The model under review builds one solid part; all positions refer to its coordinate system, in mm. A direction names the side the tool comes from. Coordinates: 2 decimals unless noted, no trailing zeros. Order: outer loops, then holes, each group sorted by start corner. A loop starts at its lowest first (then second) coordinate and runs counter-clockwise, first axis right, second up. Notation, with made-up numbers: (-24.75, 89) -> (12.25, 89) arc R11 ccw to (12.25, 93) -> close; hole circle Ø1 at (76, -19). An arc over 180 degrees is marked (long way). Put each result on its own line as item: value.
from build123d import *

# Parameters (mm, degrees)
F0_R     = 5
F1_DEPTH = 10


with BuildPart() as f1:
    # F0 (on Top) → F1 (new body)
    with BuildSketch(Plane.XY):
        with BuildLine():
            Line((-14.934364, 27.165507), (-14.585732, 20.304099))
            ThreePointArc((-14.585732, 20.304099), (-14.694631, 20.225425), (-14.803106, 20.146167))
            Line((-14.803106, 20.146167), (-21.22096, 22.598027))
            Line((-21.22096, 22.598027), (-19.176918, 16.038884))
            ThreePointArc((-19.176918, 16.038884), (-19.262831, 15.9356), (-19.348188, 15.831855))
            Line((-19.348188, 15.831855), (-26.174166, 16.610631))
            Line((-26.174166, 16.610631), (-22.563148, 10.765888))
            ThreePointArc((-22.563148, 10.765888), (-22.620676, 10.644482), (-22.677551, 10.52277))
            Line((-22.677551, 10.52277), (-29.482752, 9.579527))
            Line((-29.482752, 9.579527), (-24.531653, 4.816431))
            ThreePointArc((-24.531653, 4.816431), (-24.557181, 4.684533), (-24.582, 4.5525))
            Line((-24.582, 4.5525), (-30.938829, 1.946506))
            Line((-30.938829, 1.946506), (-24.958744, -1.43566))
            ThreePointArc((-24.958744, -1.43566), (-24.950668, -1.569763), (-24.941872, -1.70382))
            Line((-24.941872, -1.70382), (-30.450905, -5.808821))
            Line((-30.450905, -5.808821), (-23.817584, -7.597544))
            ThreePointArc((-23.817584, -7.597544), (-23.776413, -7.725425), (-23.734555, -7.853083))
            Line((-23.734555, -7.853083), (-28.049639, -13.199158))
            Line((-28.049639, -13.199158), (-21.179879, -13.282045))
            ThreePointArc((-21.179879, -13.282045), (-21.108198, -13.39567), (-21.035908, -13.508908))
            Line((-21.035908, -13.508908), (-23.885911, -19.760144))
            Line((-23.885911, -19.760144), (-17.211364, -18.131987))
            ThreePointArc((-17.211364, -18.131987), (-17.113678, -18.224216), (-17.015497, -18.315918))
            Line((-17.015497, -18.315918), (-18.221343, -25.079527))
            Line((-18.221343, -25.079527), (-12.161395, -21.84263))
            ThreePointArc((-12.161395, -21.84263), (-12.043842, -21.907667), (-11.925941, -21.972072))
            Line((-11.925941, -21.972072), (-11.411861, -28.823071))
            Line((-11.411861, -28.823071), (-6.347282, -24.180819))
            ThreePointArc((-6.347282, -24.180819), (-6.217247, -24.214579), (-6.087033, -24.24764))
            Line((-6.087033, -24.24764), (-3.88533, -30.755556))
            Line((-3.88533, -30.755556), (-0.134345, -24.999639))
            ThreePointArc((-0.134345, -24.999639), (0, -25), (0.134345, -24.999639))
            Line((0.134345, -24.999639), (3.88533, -30.755556))
            Line((3.88533, -30.755556), (6.087033, -24.24764))
            ThreePointArc((6.087033, -24.24764), (6.217247, -24.214579), (6.347282, -24.180819))
            Line((6.347282, -24.180819), (11.411861, -28.823071))
            Line((11.411861, -28.823071), (11.925941, -21.972072))
            ThreePointArc((11.925941, -21.972072), (12.043842, -21.907667), (12.161395, -21.84263))
            Line((12.161395, -21.84263), (18.221343, -25.079527))
            Line((18.221343, -25.079527), (17.015497, -18.315918))
            ThreePointArc((17.015497, -18.315918), (17.113678, -18.224216), (17.211364, -18.131987))
            Line((17.211364, -18.131987), (23.885911, -19.760144))
            Line((23.885911, -19.760144), (21.035908, -13.508908))
            ThreePointArc((21.035908, -13.508908), (21.108198, -13.39567), (21.179879, -13.282045))
            Line((21.179879, -13.282045), (28.049639, -13.199158))
            Line((28.049639, -13.199158), (23.734555, -7.853083))
            ThreePointArc((23.734555, -7.853083), (23.776413, -7.725425), (23.817584, -7.597544))
            Line((23.817584, -7.597544), (30.450905, -5.808821))
            Line((30.450905, -5.808821), (24.941872, -1.70382))
            ThreePointArc((24.941872, -1.70382), (24.950668, -1.569763), (24.958744, -1.43566))
            Line((24.958744, -1.43566), (30.938829, 1.946506))
            Line((30.938829, 1.946506), (24.582, 4.5525))
            ThreePointArc((24.582, 4.5525), (24.557181, 4.684533), (24.531653, 4.816431))
            Line((24.531653, 4.816431), (29.482752, 9.579527))
            Line((29.482752, 9.579527), (22.677551, 10.52277))
            ThreePointArc((22.677551, 10.52277), (22.620676, 10.644482), (22.563148, 10.765888))
            Line((22.563148, 10.765888), (26.174166, 16.610631))
            Line((26.174166, 16.610631), (19.348188, 15.831855))
            ThreePointArc((19.348188, 15.831855), (19.262831, 15.9356), (19.176918, 16.038884))
            Line((19.176918, 16.038884), (21.22096, 22.598027))
            Line((21.22096, 22.598027), (14.803106, 20.146167))
            ThreePointArc((14.803106, 20.146167), (14.694631, 20.225425), (14.585732, 20.304099))
            Line((14.585732, 20.304099), (14.934364, 27.165507))
            Line((14.934364, 27.165507), (9.327892, 23.194621))
            ThreePointArc((9.327892, 23.194621), (9.203114, 23.244412), (9.07807, 23.293532))
            Line((9.07807, 23.293532), (7.709387, 30.026078))
            Line((7.709387, 30.026078), (3.266571, 24.785672))
            ThreePointArc((3.266571, 24.785672), (3.133331, 24.802868), (3, 24.819347))
            Line((3, 24.819347), (0, 31))
            Line((0, 31), (-3, 24.819347))
            ThreePointArc((-3, 24.819347), (-3.133331, 24.802868), (-3.266571, 24.785672))
            Line((-3.266571, 24.785672), (-7.709387, 30.026078))
            Line((-7.709387, 30.026078), (-9.07807, 23.293532))
            ThreePointArc((-9.07807, 23.293532), (-9.203114, 23.244412), (-9.327892, 23.194621))
            Line((-9.327892, 23.194621), (-14.934364, 27.165507))
        make_face()
        with Locations((-14.526644, 0)):
            Circle(F0_R, mode=Mode.SUBTRACT)
        with BuildLine():
            ThreePointArc((17.00987, -10.519711), (0, -20), (-17.00987, -10.519711))
            ThreePointArc((-17.00987, -10.519711), (-17.014268, -8.422914), (-15.144201, -7.474532))
            ThreePointArc((-15.144201, -7.474532), (-7.026644, 0), (-15.144201, 7.474532))
            ThreePointArc((-15.144201, 7.474532), (-17.014268, 8.422914), (-17.00987, 10.519711))
            ThreePointArc((-17.00987, 10.519711), (0, 20), (17.00987, 10.519711))
            ThreePointArc((17.00987, 10.519711), (17.014268, 8.422914), (15.144201, 7.474532))
            ThreePointArc((15.144201, 7.474532), (7.026644, 0), (15.144201, -7.474532))
            ThreePointArc((15.144201, -7.474532), (17.014268, -8.422914), (17.00987, -10.519711))
        make_face(mode=Mode.SUBTRACT)
        with Locations((14.526644, 0)):
            Circle(F0_R, mode=Mode.SUBTRACT)
    extrude(amount=F1_DEPTH)


solid = f1.part
Item 1: For pin 1 Ø2 at (y, z) = (-24, 1) entering from +X; pin 2 Ø1.5 at (y, z) = (9.5, 4.5) entering from -X, all flat-tipped, find the tip position at first contact; note any pin that passes through.
Answers below:
pin 1: x = 18.21
pin 2: x = -29.48
Item 2: For line 1 (Y direction, x = 24, z = 7.75); line 2 (Y direction, x = -15.5, z = 2); line 3 (X direction, y = 3.5, z = 3), list the stretches that pass through material, from the lowest coordinate up. Write a range as from..to.
Answers below:
line 1: -13.25..-8.18, -7.55..10.34, 13.09..16.36
line 2: -23.63..-12.64, -7.48..-4.9, 4.9..7.48, 12.64..20.41
line 3: -27.15..-18.1, -10.96..-7.89, 7.89..10.96, 18.1..27.15
Item 3: Consider section D-D on z = 3.75. Count the separate pieces of the cut face and the enclosed holes in it, and give its area (3 significant figures).
Answers below:
separate pieces: 1
enclosed holes: 3
area: 1,330 mm^2
Item 4: Consider section B-B on y = -12. Write out the cut boundary in (x, z), and give its area (3 significant figures).
Answers below:
outline: (-27.08, 0) -> (-16, 0) -> (-16, 10) -> (-27.08, 10) -> close; (16, 0) -> (27.08, 0) -> (27.08, 10) -> (16, 10) -> close
area: 222 mm^2
Item 5: Consider section C-C on y = 0. Write out the cut boundary in (x, z).
Answers below:
outline: (-27.5, 0) -> (-19.53, 0) -> (-19.53, 10) -> (-27.5, 10) -> close; (-9.53, 0) -> (-7.03, 0) -> (-7.03, 10) -> (-9.53, 10) -> close; (7.03, 0) -> (9.53, 0) -> (9.53, 10) -> (7.03, 10) -> close; (19.53, 0) -> (27.5, 0) -> (27.5, 10) -> (19.53, 10) -> close
Item 6: Consider section A-A on x = -1. Write out the cut boundary in (y, z).
Answers below:
outline: (-26.33, 0) -> (-19.97, 0) -> (-19.97, 10) -> (-26.33, 10) -> close; (19.97, 0) -> (28.94, 0) -> (28.94, 10) -> (19.97, 10) -> close
Item 7: Mouldability with a two-part tool opening along X and no side actions: class faces 5 (the flat face through (-25.862, -10.489, 4.93)), 6 (the flat face through (1.52, 27.87, 4.93)), 7 (the cylindrical face through (0, 20, 5)), 8 (the flat face through (-7.3, 0.6, 0)) as +X half, -X half, draft (parallel to the pull), parting line (faces both ways), or undercut.
Answers below:
face 5: -X half
face 6: undercut
face 7: undercut
face 8: draft
Item 8: For faces 1 (the flat face through (8.403, 26.613, 4.93)), 2 (the flat face through (24.343, 13.647, 4.93)), 3 (the flat face through (4.97, -27.55, 4.93)), 4 (the flat face through (-22.44, -16.59, 4.93)), list the 3-axis set-ups (+Z, -Z, +X, -X, +Y, -Y) from which the entire face can be reached by the end or side of a thin tool; tool diameter is ignored.
Answers below:
face 1: +Z, -Z, +Y
face 2: +Z, -Z, +X
face 3: +Z, -Z, -Y
face 4: +Z, -Z, -X
